Geometry: see drawing. Coordinates: mm, zero at the bounding-box minimum. Round coordinates to 2 decimals unless told otherwise and drop trailing zeros. Order: outer loops, then holes, each group sorted by start corner. A loop starts at its lowest first (then second) coordinate and runs counter-clockwise, first axis right, second up. Notation, with made-up numbers: M 80,73 L 84,73 A32 cw 84,111 Z; hole C -37,42 d10. An arc over 180 degrees is marked long. Answer in a Markdown table with one row per item. Add a question column.
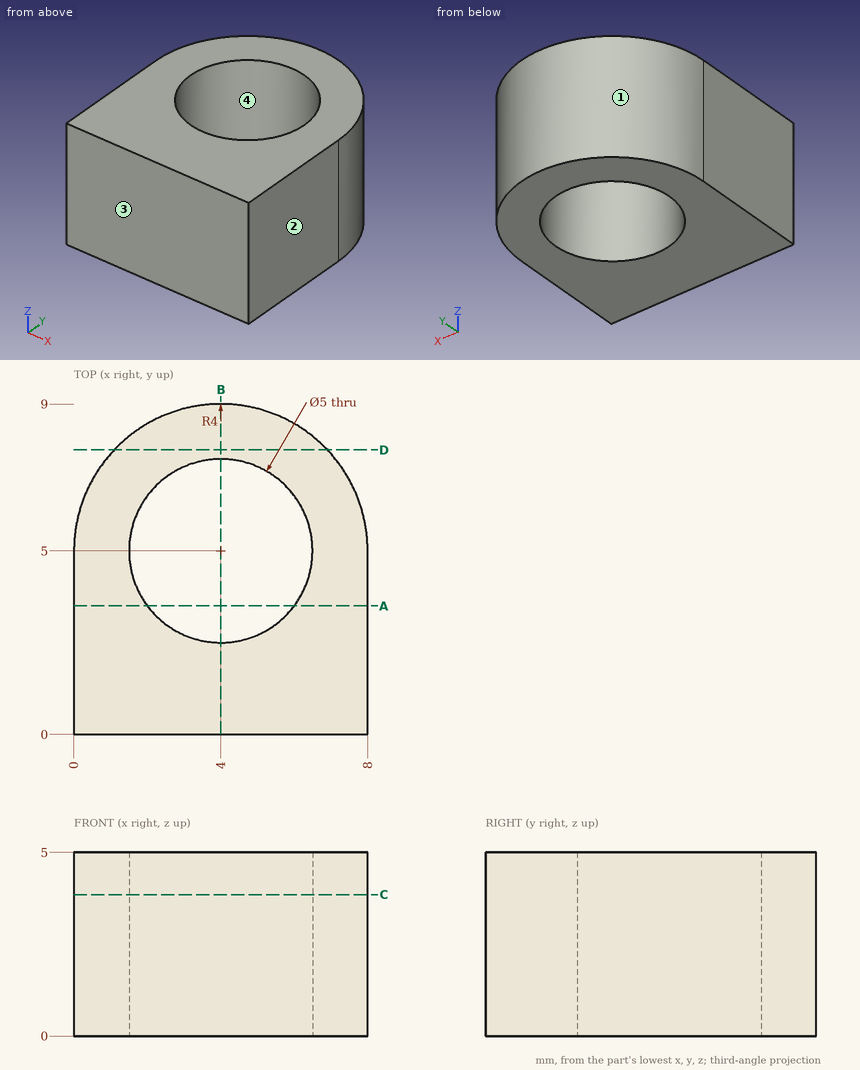
(1) Cut plane C-C (z = 3.85). Return loops of the section in (x, y), and give its area (3 significant figures).
(2) Draft query along Y for the marked faces 1, 2, 3 and 4. Return one class per face: +Y half, -Y half, draft (parallel to the pull), parting line (faces both ways), or undercut.
(3) Line query: line 1 (Y direction, x = 4, z = 2.5); line 2 (X direction, y = 7, z = 2); line 3 (X direction, y = 5.25, z = 3.2). Output: solid intervals per line, ascending. Write a range as from..to.
(4) Cut plane B-B (x = 4). Return loops of the section in (y, z), and give its area (3 significant figures).
(5) Cut plane A-A (y = 3.5). Return loops of the section in (x, z).
(6) Cut plane D-D (y = 7.75). Return loops of the section in (x, z).
Answer list:
| question | item | result |
|---|---|---|
| 1 | outline | M 0,0 L 8,0 L 8,5 A4 ccw 0,5 Z; hole C 4,5 d5 |
| 1 | area | 45.5 mm² |
| 2 | face 1 | +Y half |
| 2 | face 2 | draft |
| 2 | face 3 | -Y half |
| 2 | face 4 | undercut |
| 3 | line 1 | 0..2.5, 7.5..9 |
| 3 | line 2 | 0.54..2.5, 5.5..7.46 |
| 3 | line 3 | 0.01..1.51, 6.49..7.99 |
| 4 | outline | M 0,0 L 2.5,0 L 2.5,5 L 0,5 Z; M 7.5,0 L 9,0 L 9,5 L 7.5,5 Z |
| 4 | area | 20.0 mm² |
| 5 | outline | M 0,0 L 2,0 L 2,5 L 0,5 Z; M 6,0 L 8,0 L 8,5 L 6,5 Z |
| 6 | outline | M 1.1,0 L 6.9,0 L 6.9,5 L 1.1,5 Z |
